Can you work these out from the drawing? Everything is in mm from the part's minimum corner. A direction names the side the tool comes from. Give positions to 0.01 mm unless a question says otherwise; leave off trailing zeros. Order: outer loops, then holes, each group sorted by start corner. A loop starts at its lowest first (then second) coordinate and runs counter-clockwise, first axis right, second up. Notation, with made-up numbers: M -39,21.5 L 4,21.5 A19 cw 4,39.5 Z; hole C 80.25,23 d2. An arc over 180 degrees is marked long. Use a Markdown table: item, result. Add a question column.
Item 1: Suppose I cut it at D-D on x = 4.25. Write out the boundary of the cut face in (y, z).
Item 2: If we mould it in two halves opening along Y, with no side actions, what happens to the marked faces 1, 2 and 3? For each: released by +Y, released by -Y, zero draft, split by the parting line, or undercut.
Item 3: Suppose I cut it at A-A on y = 5. Write out the boundary of the cut face in (x, z).
Item 4: Suppose I cut it at C-C on z = 8.25. Write out the boundary of the cut face in (x, y) (1 decimal).
Item 5: Suppose I cut it at B-B on x = 9. Write out the boundary of the cut face in (y, z), plus the area to 3 significant figures.
Item 6: If I drill on L1, parallel to X at y = 2.75, z = 3.25; L2, parallel to Y at x = 5.5, z = 4.25; L3, parallel to X at y = 6.5, z = 6.75 (1 decimal), over which ranges is the centre line in solid material (lowest first)? Write a range as from..to.
Item 7: For the marked faces 4 and 5, which set-ups out of +Z, -Z, +X, -X, +Y, -Y let a thin tool reach every point of the face, with its end or its side?
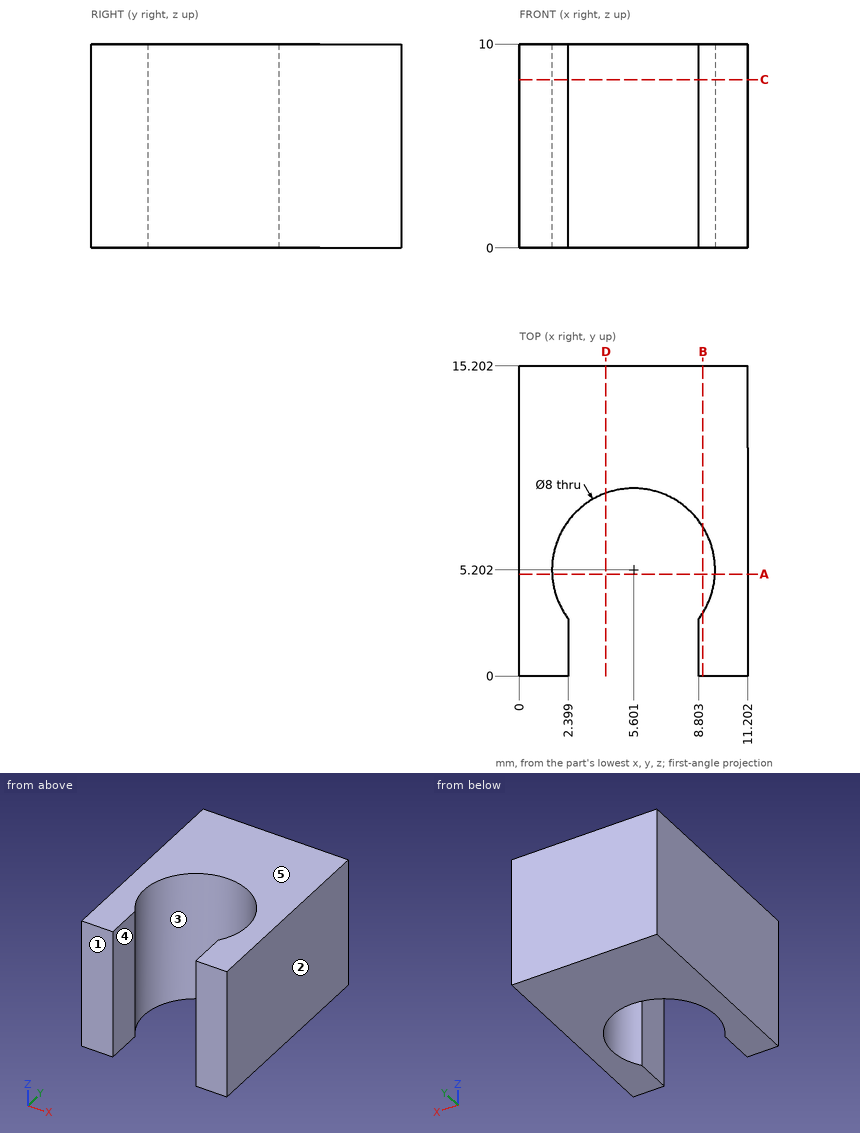
Findings below:
| question | item | result |
|---|---|---|
| 1 | outline | M 8.97,0 L 15.2,0 L 15.2,10 L 8.97,10 Z |
| 2 | face 1 | released by -Y |
| 2 | face 2 | zero draft |
| 2 | face 3 | undercut |
| 3 | outline | M 0,0 L 1.61,0 L 1.61,10 L 0,10 Z; M 9.6,0 L 11.2,0 L 11.2,10 L 9.6,10 Z |
| 4 | outline | M 0,0 L 2.4,0 L 2.4,2.8 A4 cw long 8.8,2.8 L 8.8,0 L 11.2,0 L 11.2,15.2 L 0,15.2 Z |
| 5 | outline | M 0,0 L 3.09,0 L 3.09,10 L 0,10 Z; M 7.31,0 L 15.2,0 L 15.2,10 L 7.31,10 Z |
| 5 | area | 110 mm^2 |
| 6 | L1 | x = 0..2.4, 8.8..11.2 |
| 6 | L2 | y = 9.2..15.2 |
| 6 | L3 | x = 0..1.8, 9.4..11.2 |
| 7 | face 4 | +Z, -Z, -Y |
| 7 | face 5 | +Z, +X, -X, +Y, -Y |
